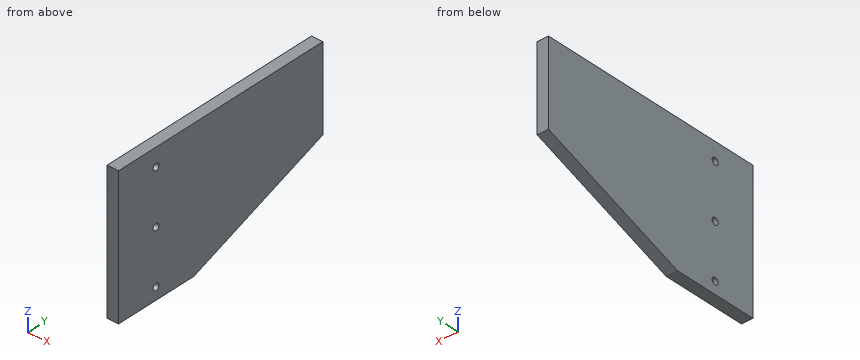
```python
from build123d import *

# Parameters (mm, degrees)
SKETCH1_R           = 3.571875
BOSS_EXTRUDE1_DEPTH = 11.90625


with BuildPart() as part:
    # Sketch1 → Boss-Extrude1 (new body)
    with BuildSketch(Plane(origin=(0, 0, 0), x_dir=(0, 0, -1), z_dir=(1, 0, 0))):
        Polygon((0, 0), (0, 241.3), (88.9, 241.3), (146.05, 88.9), (146.05, 0), align=None)
        with Locations((19.05, 44.45)):
            Circle(SKETCH1_R, mode=Mode.SUBTRACT)
        with Locations((76.2, 44.45)):
            Circle(SKETCH1_R, mode=Mode.SUBTRACT)
        with Locations((133.35, 44.45)):
            Circle(SKETCH1_R, mode=Mode.SUBTRACT)
    extrude(amount=BOSS_EXTRUDE1_DEPTH)


solid = part.part
```
Here's how the part is built. I have some questions about the finished solid (model axes, mm). Give positions to 0.01 mm unless a question says otherwise; leave off trailing zeros. Write each loop counter-clockwise with the first axis right and the second up, starting at its lowest first coordinate (ties: lowest second). Pieces come first, ordered by that corner, then holes.
(1) Imagine slicing it at D-D, the plane z = -133.35. Write out the boundary of the cut face in (x, y), and give its area (3 significant figures).
Output values:
outline: (0, 0) - (11.91, 0) - (11.91, 40.88) - (0, 40.88) - close; (0, 48.02) - (11.91, 48.02) - (11.91, 122.77) - (0, 122.77) - close
area: 1,380 mm2
(2) Will these pins go through, and if not, where does the flat tip stop? pin 1 (4 mm diameter, centred on x = 6, y = 176, fed in from -Z); pin 2 (4.5 mm diameter, centred on y = 44.45, z = -76.2, fed in from -X).
Output values:
pin 1: stops at z = -114.14
pin 2: passes through
(3) If I drill on L1, parallel to Y at x = 8.5, z = -76.2; L2, parallel to Y at x = 3.5, z = -79; L3, parallel to Z at x = 1, y = 103.5 (3 decimals), over which ranges is the centre line in solid material (lowest first)?
Output values:
L1: y = 0 to 40.88, 48.02 to 241.3
L2: y = 0 to 42.23, 46.67 to 241.3
L3: z = -140.575 to 0
(4) Imagine slicing it at B-B, the plane y = 44.45. Write out the boundary of the cut face in (x, z).
Output values:
outline: (0, -146.05) - (11.91, -146.05) - (11.91, -136.92) - (0, -136.92) - close; (0, -129.78) - (11.91, -129.78) - (11.91, -79.77) - (0, -79.77) - close; (0, -72.63) - (11.91, -72.63) - (11.91, -22.62) - (0, -22.62) - close; (0, -15.48) - (11.91, -15.48) - (11.91, 0) - (0, 0) - close
(5) Imagine slicing it at C-C, the plane x = 4.5. Write out the boundary of the cut face in (y, z).
Output values:
outline: (0, -146.05) - (88.9, -146.05) - (241.3, -88.9) - (241.3, 0) - (0, 0) - close; hole circle Ø7.14 at (44.45, -133.35); hole circle Ø7.14 at (44.45, -76.2); hole circle Ø7.14 at (44.45, -19.05)
(6) Imagine slicing it at A-A, the plane z = -19.05. Write out the boundary of the cut face in (x, y), and give its area (3 significant figures).
Output values:
outline: (0, 0) - (11.91, 0) - (11.91, 40.88) - (0, 40.88) - close; (0, 48.02) - (11.91, 48.02) - (11.91, 241.3) - (0, 241.3) - close
area: 2,790 mm2
